from build123d import *

# Parameters (mm, degrees)
SKETCH1_R           = 3.5
BOSS_EXTRUDE1_DEPTH = 3
CUT_EXTRUDE1_DEPTH  = 0.2


with BuildPart() as part:
    # Sketch1 → Boss-Extrude1 (new body)
    with BuildSketch(Plane.XY):
        Circle(SKETCH1_R)
    extrude(amount=BOSS_EXTRUDE1_DEPTH)

    # Sketch2 → Cut-Extrude1 (cut)
    with BuildSketch(Plane.XY.offset(3)):
        with BuildLine():
            Line((-0.781290974, 1.669629579), (-0.098398346, 1.669629579))
            add(Edge.make_bspline(
                [(-0.098398346, 1.669629579), (-0.064969868, 1.669453828), (-0.000177158, 1.66911318), (0.094042284, 1.663830049), (0.182291095, 1.656626379), (0.264594867, 1.645196287), (0.34091557, 1.63140451), (0.411483207, 1.614702693), (0.476073379, 1.59467608), (0.553186116, 1.562829799), (0.641106776, 1.51550663), (0.736305169, 1.445578065), (0.817709408, 1.360045602), (0.887895726, 1.263562947), (0.943696845, 1.157427175), (0.984066143, 1.044167986), (1.009624018, 0.925246244), (1.012252452, 0.843603066), (1.013580821, 0.802341919)],
                knots=[0, 0, 0, 0, 0.00010027, 0.000194349, 0.000283026, 0.000365821, 0.000443519, 0.000515622, 0.000583254, 0.00064614, 0.000765662, 0.000881909, 0.000998927, 0.001118415, 0.001238844, 0.00135727, 0.001478274, 0.001601912, 0.001601912, 0.001601912, 0.001601912], degree=3))
            add(Edge.make_bspline(
                [(1.013580821, 0.802341919), (1.012487602, 0.763689363), (1.010339325, 0.687733446), (0.989796565, 0.576639337), (0.957635897, 0.470888118), (0.912930648, 0.370865732), (0.854828652, 0.278832119), (0.785970333, 0.194044853), (0.70289353, 0.120093796), (0.64065029, 0.078750894), (0.609033545, 0.057750572)],
                knots=[0, 0, 0, 0, 0.000115857, 0.00022767, 0.000337672, 0.000446877, 0.000555233, 0.000663318, 0.000773539, 0.000887324, 0.000887324, 0.000887324, 0.000887324], degree=3))
            add(Edge.make_bspline(
                [(0.609033545, 0.057750572), (0.648793972, 0.042485573), (0.72486552, 0.013279849), (0.829551532, -0.038355615), (0.919746377, -0.094517725), (0.996143523, -0.155849575), (1.061481178, -0.221958386), (1.11853412, -0.293813501), (1.167215494, -0.372352258), (1.208928417, -0.456755794), (1.241477174, -0.546162262), (1.265853078, -0.639733038), (1.279820527, -0.737132593), (1.281808168, -0.803417973), (1.28281159, -0.836880838)],
                knots=[0, 0, 0, 0, 0.000127722, 0.000244363, 0.000349599, 0.000445847, 0.000537565, 0.000627901, 0.000720503, 0.000814257, 0.000909859, 0.001005428, 0.001103887, 0.001204268, 0.001204268, 0.001204268, 0.001204268], degree=3))
            add(Edge.make_bspline(
                [(1.28281159, -0.836880838), (1.281834744, -0.87104771), (1.279912772, -0.938271988), (1.2657328, -1.037027123), (1.241723693, -1.131402069), (1.208652547, -1.222007252), (1.165490232, -1.308667386), (1.112962268, -1.39148065), (1.050330704, -1.469614981), (0.980267835, -1.543938604), (0.90100569, -1.610766391), (0.815489935, -1.670282098), (0.722643615, -1.71922816), (0.623991621, -1.760344182), (0.518427305, -1.79175138), (0.406424697, -1.813723954), (0.288080396, -1.828528991), (0.206870644, -1.829746196), (0.165223449, -1.830370421)],
                knots=[0, 0, 0, 0, 0.000102481, 0.000201635, 0.000298562, 0.000394165, 0.000490425, 0.000588455, 0.000687769, 0.000790423, 0.000894381, 0.000998232, 0.001102369, 0.001208616, 0.001318415, 0.001432129, 0.001550749, 0.00167562, 0.00167562, 0.00167562, 0.00167562], degree=3))
            Line((0.165223449, -1.830370421), (-0.781290974, -1.830370421))
            Line((-0.781290974, -1.830370421), (-0.781290974, 1.669629579))
        make_face()
        with BuildLine():
            Line((-0.46718841, 1.31065522), (-0.46718841, 0.188860348))
            Line((-0.46718841, 0.188860348), (-0.25615075, 0.188860348))
            add(Edge.make_bspline(
                [(-0.25615075, 0.188860348), (-0.225301955, 0.189260271), (-0.165695795, 0.190033004), (-0.079375899, 0.192246521), (0.000749119, 0.198444564), (0.074540952, 0.204640826), (0.141883396, 0.214715414), (0.202627258, 0.226707537), (0.257725855, 0.239390442), (0.3212654, 0.260959929), (0.393338349, 0.292837604), (0.470171453, 0.34230944), (0.537905923, 0.401233793), (0.59510311, 0.469224755), (0.641914581, 0.544090941), (0.674428296, 0.624637821), (0.69647558, 0.708857953), (0.698467112, 0.766676206), (0.699478256, 0.796031822)],
                knots=[0, 0, 0, 0, 9.2559e-05, 0.000178842, 0.000258967, 0.000333616, 0.000400942, 0.000463093, 0.000519379, 0.000570374, 0.000664201, 0.000755025, 0.000843472, 0.000932526, 0.001020669, 0.001107124, 0.001192318, 0.001280185, 0.001280185, 0.001280185, 0.001280185], degree=3))
            add(Edge.make_bspline(
                [(0.699478256, 0.796031822), (0.698952076, 0.815457594), (0.697919916, 0.853563366), (0.689466614, 0.90911272), (0.675099039, 0.961356473), (0.656644746, 1.011010583), (0.630856057, 1.056522433), (0.600492594, 1.099465629), (0.563806904, 1.138377747), (0.522049591, 1.174747246), (0.474040968, 1.206991774), (0.419809676, 1.235232537), (0.358621999, 1.257973313), (0.291509144, 1.277889466), (0.217438057, 1.29187776), (0.137263503, 1.303531147), (0.050328784, 1.309463889), (-0.009816318, 1.310249252), (-0.040906359, 1.31065522)],
                knots=[0, 0, 0, 0, 5.8261e-05, 0.000114285, 0.000168029, 0.000220632, 0.000272728, 0.000324483, 0.000378062, 0.000432741, 0.000490301, 0.000551137, 0.000615721, 0.000685833, 0.000760908, 0.00084162, 0.000928788, 0.00102206, 0.00102206, 0.00102206, 0.00102206], degree=3))
            Line((-0.040906359, 1.31065522), (-0.46718841, 1.31065522))
        make_face(mode=Mode.SUBTRACT)
        with BuildLine():
            Line((-0.46718841, -0.170114011), (-0.46718841, -1.471396062))
            Line((-0.46718841, -1.471396062), (-0.019872705, -1.471396062))
            add(Edge.make_bspline(
                [(-0.019872705, -1.471396062), (0.012146221, -1.471012315), (0.073858479, -1.470272692), (0.16295971, -1.467858138), (0.245542813, -1.462365862), (0.321230949, -1.453720012), (0.390841402, -1.444341563), (0.453539105, -1.431730282), (0.509832298, -1.417281322), (0.575106606, -1.39494715), (0.648610114, -1.360250679), (0.727820971, -1.307936452), (0.798247189, -1.245613144), (0.858052448, -1.17348223), (0.907065436, -1.095050903), (0.942720892, -1.011905553), (0.964711748, -0.925420026), (0.967373918, -0.866453313), (0.968709026, -0.836880838)],
                knots=[0, 0, 0, 0, 9.6064e-05, 0.000185151, 0.000267373, 0.000344257, 0.000413665, 0.000478015, 0.000536005, 0.000587888, 0.000684801, 0.000778918, 0.000871787, 0.000965866, 0.001059062, 0.00114827, 0.001236355, 0.001324974, 0.001324974, 0.001324974, 0.001324974], degree=3))
            add(Edge.make_bspline(
                [(0.968709026, -0.836880838), (0.968432921, -0.818387497), (0.967885166, -0.781699116), (0.959624551, -0.727783296), (0.947610682, -0.675557423), (0.932079248, -0.624879683), (0.909459781, -0.576666306), (0.883053236, -0.529963747), (0.852091834, -0.484710267), (0.803847668, -0.427498014), (0.733675683, -0.361581001), (0.633968908, -0.297043499), (0.52059661, -0.244995692), (0.438369117, -0.222896215), (0.395892519, -0.211480197)],
                knots=[0, 0, 0, 0, 5.5429e-05, 0.000109963, 0.000163198, 0.000216191, 0.000268588, 0.000322593, 0.000377046, 0.000432793, 0.000546889, 0.000664343, 0.000787646, 0.000919405, 0.000919405, 0.000919405, 0.000919405], degree=3))
            add(Edge.make_bspline(
                [(0.395892519, -0.211480197), (0.378863423, -0.208025113), (0.341940831, -0.200533778), (0.281733251, -0.192626075), (0.212997382, -0.185581015), (0.135574504, -0.180369857), (0.049366663, -0.174983314), (-0.045810255, -0.172888493), (-0.14956757, -0.170389233), (-0.221559942, -0.170208098), (-0.258955237, -0.170114011)],
                knots=[0, 0, 0, 0, 5.2115e-05, 0.000112995, 0.000182062, 0.000259389, 0.000345767, 0.00044116, 0.000544948, 0.000657129, 0.000657129, 0.000657129, 0.000657129], degree=3))
            Line((-0.258955237, -0.170114011), (-0.46718841, -0.170114011))
        make_face(mode=Mode.SUBTRACT)
    extrude(amount=-CUT_EXTRUDE1_DEPTH, mode=Mode.SUBTRACT)


solid = part.part
Input: part model. Units: mm. Frame: model coordinates. Coordinates: 2 decimals unless noted, no trailing zeros. Order: outer loops, then holes, each group sorted by start corner. A loop starts at its lowest first (then second) coordinate and runs counter-clockwise, first axis right, second up. Notation, with made-up numbers: M 56.25,-18.5 L 78.25,-18.5 A30 cw 78.25,17.5 Z; hole C -20,-4.75 d8. An arc over 180 degrees is marked long. One line per question, with ' | ' between items.
Item 1: Section A-A (x = -1.5). Output: boundary loops of the cut face in (y, z), then the cut area to 3 significant figures.
Geometry results:
outline: M -3.16,0 L 3.16,0 L 3.16,3 L -3.16,3 Z | area: 19.0 mm^2
Item 2: Section B-B (z = 1.9). Output: boundary loops of the cut face in (x, y).
Geometry results:
outline: C 0,0 d7
Item 3: Draft query along Y for faces 1 (the cylindrical face through (3.233, -1.341, 1.479)), 2 (the flat face through (0, -1, 3)), 3 (the flat face through (0, 0, 2.8)). Return one class per face: released by +Y, released by -Y, zero draft, split by the parting line, or undercut.
Geometry results:
face 1: split by the parting line | face 2: zero draft | face 3: undercut
Item 4: Ray query, line 1 along X through (y, z) = (-2.5, 0.6); line 2 along X through (y, z) = (-3, 2.1); line 3 along Y through (x, z) = (-1.25, 2.05). Return the intervals inside material, ascending.
Geometry results:
line 1: x = -2.45 to 2.45 | line 2: x = -1.8 to 1.8 | line 3: y = -3.27 to 3.27
Item 5: Section C-C (y = -2.5). Output: boundary loops of the cut face in (x, z).
Geometry results:
outline: M -2.45,0 L 2.45,0 L 2.45,3 L -2.45,3 Z
